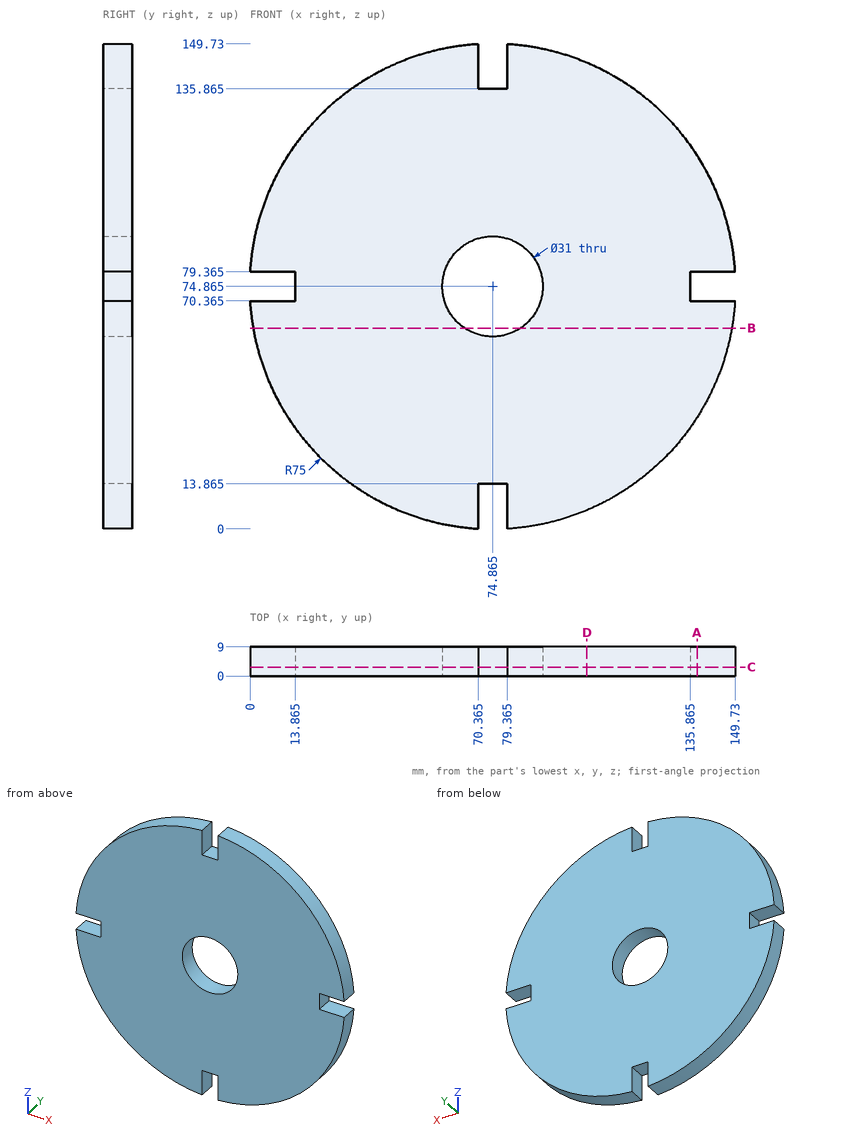
Can you work these out from the drawing? Everything is in mm from the part's minimum corner. Round coordinates to 2 decimals unless told otherwise and drop trailing zeros. Write each loop counter-clockwise with the first axis right and the second up, starting at its lowest first coordinate (ties: lowest second). Pieces come first, ordered by that corner, then holes. Notation, with made-up numbers: M 35,58.25 L 42,58.25 A25 cw 42,94.25 Z; hole C 41,79.25 d10. An arc over 180 degrees is marked long. Use a Markdown table: item, result.
Item 1: I want a section at D-D (x = 104). List the corners of the cut face in (y, z) for me (1 decimal), and give its area (3 significant figures).
Found:
| item | result |
|---|---|
| outline | M 0,5.8 L 9,5.8 L 9,144 L 0,144 Z |
| area | 1,240 mm2 |
Item 2: I want a section at A-A (x = 138). List the corners of the cut face in (y, z) for me (1 decimal).
Found:
| item | result |
|---|---|
| outline | M 0,34.4 L 9,34.4 L 9,70.4 L 0,70.4 Z; M 0,79.4 L 9,79.4 L 9,115.3 L 0,115.3 Z |
Item 3: For pin 1 Ø1 at (x, y) = (92.5, 1.5) entering from +Z; pin 2 Ø4.5 at (y, z) = (6, 6.5) entering from +X (1 decimal); pin 3 Ø2.5 at (y, z) = (4, 143.5) entering from +X, each with a flat end and sliding along its axis, tell me the tip position at first contact or that it passes through.
Found:
| item | result |
|---|---|
| pin 1 | stops at z = 147.88 |
| pin 2 | stops at x = 110.3 |
| pin 3 | stops at x = 107.79 |
Item 4: If I drill on line 1 along Z through (x, y) = (13, 7) (1 decimal); line 2 along Z through (x, y) = (77, 8.5) (1 decimal); line 3 along X through (y, z) = (3, 82.5) (1 decimal), over which ranges is the centre line in solid material (lowest first)? Write a range as [from, to].
Found:
| item | result |
|---|---|
| line 1 | z = [32.5, 70.4], [79.4, 117.3] |
| line 2 | z = [13.9, 59.5], [90.2, 135.9] |
| line 3 | x = [0.3, 61.4], [88.4, 149.5] |
Item 5: I want a section at C-C (y = 2.75). List the corners of the cut face in (x, z) for me (1 decimal), and give its area (3 significant figures).
Found:
| item | result |
|---|---|
| outline | M 0,70.4 A75 ccw 70.4,0 L 70.4,13.9 L 79.4,13.9 L 79.4,0 A75 ccw 149.7,70.4 L 135.9,70.4 L 135.9,79.4 L 149.7,79.4 A75 ccw 79.4,149.7 L 79.4,135.9 L 70.4,135.9 L 70.4,149.7 A75 ccw 0,79.4 L 13.9,79.4 L 13.9,70.4 Z; hole C 74.9,74.9 d31 |
| area | 16,400 mm2 |
Item 6: I want a section at B-B (z = 62). List the corners of the cut face in (x, y) for me, and give its area (3 significant figures).
Found:
| item | result |
|---|---|
| outline | M 0.98,0 L 66.22,0 L 66.22,9 L 0.98,9 Z; M 83.51,0 L 148.75,0 L 148.75,9 L 83.51,9 Z |
| area | 1,170 mm2 |
